```python
from build123d import *

# Parameters (mm, degrees)
SKETCH1_R                = 25
BOSS_EXTRUDE1_DEPTH      = 400
BOSS_EXTRUDE2_DEPTH      = 10
BOSS_EXTRUDE2_DEPTH_BACK = 10
SKETCH2_R                = 15
CUT_EXTRUDE1_START       = -70
SKETCH3_R                = 32.241288232
SKETCH3_R_2              = 25
CUT_EXTRUDE1_DEPTH       = 70


with BuildPart() as part:
    # Sketch1 → Boss-Extrude1 (new body)
    with BuildSketch(Plane(origin=(0, 0, 0), x_dir=(0, 0, -1), z_dir=(1, 0, 0))):
        Circle(SKETCH1_R)
    extrude(amount=BOSS_EXTRUDE1_DEPTH)

    # Sketch2 → Boss-Extrude2 (add, two sides: drawn at the far end of the back side and taken through both)
    with BuildSketch(Plane.XY.offset(-BOSS_EXTRUDE2_DEPTH_BACK)):
        with BuildLine():
            Line((0, 25), (0, -25))
            Line((0, -25), (-35, -20))
            ThreePointArc((-35, -20), (-55, 0), (-35, 20))
            Line((-35, 20), (0, 25))
        make_face()
        with Locations((-35, 0)):
            Circle(SKETCH2_R, mode=Mode.SUBTRACT)
    extrude(amount=BOSS_EXTRUDE2_DEPTH + BOSS_EXTRUDE2_DEPTH_BACK)

    # Sketch3 → Cut-Extrude1 (cut)
    with BuildSketch(Plane(origin=(0, 0, 0), x_dir=(0, 0, -1), z_dir=(1, 0, 0)).offset(CUT_EXTRUDE1_START)):
        Circle(SKETCH3_R)
        with Locations(Location((0, 0, 0), (0, 0, 113.578178478))):
            Circle(SKETCH3_R_2, mode=Mode.SUBTRACT)
    extrude(amount=CUT_EXTRUDE1_DEPTH, mode=Mode.SUBTRACT)


solid = part.part
```
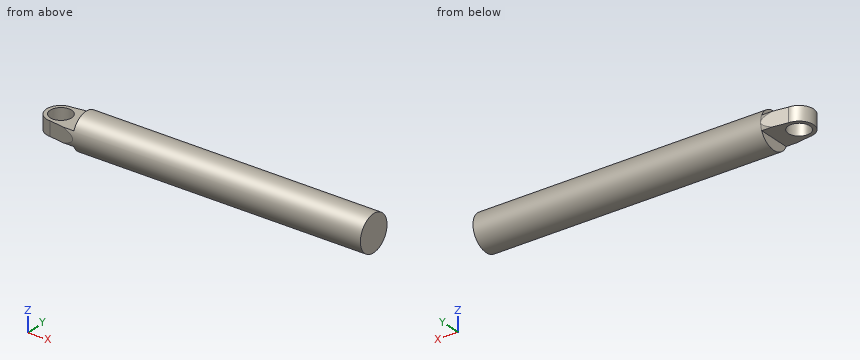
Input: part model. Units: mm. Frame: model coordinates. Give positions to 0.01 mm unless a question says otherwise; leave off trailing zeros. Order: outer loops, then holes, each group sorted by start corner. A loop starts at its lowest first (then second) coordinate and runs counter-clockwise, first axis right, second up.
1. Section B-B on x = 173. Return the cut outline in (y, z), and give its area (3 significant figures).
Derived:
outline: circle Ø50 at (0, 0)
area: 1,960 mm2
2. Section C-C on z = 14.5. Return the cut outline in (x, y), and give its area (3 significant figures).
Derived:
outline: (0, -20.37) - (400, -20.37) - (400, 20.37) - (0, 20.37) - close
area: 16,300 mm2
3. Section D-D on z = -17. Return the cut outline in (x, y).
Derived:
outline: (0, -18.33) - (400, -18.33) - (400, 18.33) - (0, 18.33) - close
4. Material intervals for L1, parallel to Y at x = -35, z = -3; L2, parallel to X at y = -1.5, z = 0; L3, parallel to X at y = 1, z = 8, sorted ascending.
Derived:
L1: y = -20 to -15, 15 to 20
L2: x = -54.94 to -49.92, -20.08 to 400
L3: x = -54.97 to -49.97, -20.03 to 400
5. Pin query (flat end, axial travel): pin 1 (10 mm diameter, centred on y = -12.5, z = -2.5, fed in from -X); pin 2 (12 mm diameter, centred on x = 315, y = 15.5, fed in from -Z); pin 3 (10 mm diameter, centred on x = 107, y = -8.5, fed in from +Z). Return the tip coordinate at first contact, or that it passes through.
Derived:
pin 1: stops at x = -53.54
pin 2: stops at z = -23.12
pin 3: stops at z = 24.75
6. Section A-A on y = 0. Return the cut outline in (x, z).
Derived:
outline: (-55, -10) - (-50, -10) - (-50, 10) - (-55, 10) - close; (-20, -10) - (0, -10) - (0, -25) - (400, -25) - (400, 25) - (0, 25) - (0, 10) - (-20, 10) - close
